Autodesk Inventor part; units mm, degrees
ref_plane "YZ Plane" through (0, 0, 0) normal (1, 0, 0) x (0, 1, 0)
ref_plane "XZ Plane" through (0, 0, 0) normal (0, 1, 0) x (-1, 0, 0)
ref_plane "XY Plane" through (0, 0, 0) normal (0, 0, 1) x (1, 0, 0)
sketch "Skizze1" plane through (0, 0, 0) normal (0, 0, 1) x (1, 0, 0)
  line L0 (21, -21) -> (-21, -21)
  line L1 (-21, -21) -> (-21, 21)
  line L2 (-21, 21) -> (21, 21)
  line L3 (21, 21) -> (21, -21)
  line L4 (21, -21) -> (-21, 21) construction
  line L5 (-21, -21) -> (21, 21) construction
  circle A0 centre (0, 0) radius 18
  circle A1 centre (-15.5, 15.5) radius 1.6
  circle A2 centre (15.5, 15.5) radius 1.6
  circle A3 centre (15.5, -15.5) radius 1.6
  circle A4 centre (-15.5, -15.5) radius 1.6
  dimension "d0" = 42
  dimension "d1" = 42
  dimension "d2" = 36
  dimension "d3" = 31
  dimension "d4" = 15.5
  dimension "d5" = 3.2
  dimension "d6" = 3.2
  dimension "d7" = 3.2
  dimension "d8" = 3.2
extrude "Extrusion1" add sketch "Skizze1" along normal blind 20
sketch "Skizze2" plane through (21, -21, 0) normal (1, 0, 0) x (0, 0, -1)
  line L0 (-25, -16) -> (5, -16)
  line L1 (5, -16) -> (5, 58)
  line L2 (5, 58) -> (-25, 58)
  line L3 (-25, 58) -> (-25, -16)
  line L4 (-25, -16) -> (5, 58) construction
  line L5 (5, -16) -> (-25, 58) construction
  line L6 (0, 0) -> (-20, 0)
  line L7 (0, 42) -> (-20, 42)
  line L8 (0, 42) -> (0, 0)
  point P0 (0, 21)
  point P1 (-10, 21)
  point P2 (0, 21)
  dimension "d11" = 30
  dimension "d12" = 74
  dimension "d13" = 42
  dimension "d14" = 20
  dimension "d15" = 10
  dimension "d16" = 21
extrude "Extrusion2" add sketch "Skizze2" along normal blind 4
sketch "Skizze3" plane through (21, -21, 0) normal (-1, 0, 0) x (0, 0, 1)
  line L0 (0, 0) -> (20, 0)
  line L1 (25, -16) -> (-5, -16)
  line L2 (25, 58) -> (25, -16)
  point P0 (0, 21)
  point P1 (10, -8)
  dimension "d19" = 16
  dimension "d20" = 15
  dimension "d21" = 30
  dimension "d22" = 8
hole "Bohrung1" at (21, -29, 10) direction (1, 0, 0) diameter 5.5 end through all counterbore diameter 15 counterbore depth 1
ref_plane "Arbeitsebene1" through (21, 0, -5) normal (0, -1, 0) x (0, 0, -1)
mirror "Spiegeln1" about plane through (21, 0, -5) normal (0, -1, 0) of "Bohrung1"
chamfer "Fase1" distance 4 angle 45 2 edges at (-21, -21, 10) (-21, 21, 10)
fillet "Rundung1" radius 2 4 edges at (21, 0, 20) (21, -21, 10) (21, 21, 10) (21, 0, 0)
fillet "Rundung2" radius 3 2 edges at (21, -37, 10) (21, 37, 10)
chamfer "Fase2" distance 1 angle 45 10 edges at (21, 0, 25) (21.8787, -36.1213, 25) (24.5, -37, 25) (21.8787, 36.1213, 25) (24.5, 37, 25) (21, 0, -5) (21.8787, 36.1213, -5) (24.5, 37, -5) (21.8787, -36.1213, -5) (24.5, -37, -5)
chamfer "Fase3" distance 1 angle 45 2 edges at (-18, 0, 20) (-18, 0, 0)
equation "\"d1\" = d0"
equation "\"d6\" = d5"
properties part number "bullog_mount"
Can you work these out from the model? Positions are in its coordinate system, mm. A direction names the side the tool comes from. Coordinates: 2 decimals unless noted, no trailing zeros. Loops run counter-clockwise (first coordinate to the right, second up) from the corner with the lowest first, then second, coordinate; pieces in that order, holes last. Notation, with made-up numbers: (9, 17.25) - (53, 17.25) arc R22 cw to (53, 46.25) - close; hole circle Ø2 at (69, 37). An arc over 180 degrees is marked (long way). Answer as a JSON object with one key per item and string values. Group by question number.
Item 1: If we section it at D-D (x = 15.5): State how many separate pieces and enclosed holes the cut face has, plus the area to 3 significant figures.
Item 2: If we section it at C-C (z = 6.5): List the corners of the cut face in (x, y) for me.
Item 3: For pin 1 (4 mm diameter, centred on x = 17.5, z = 11.5, fed in from +Y); pin 2 (4.5 mm diameter, centred on y = 26.5, z = 13, fed in from -X); pin 3 (1.5 mm diameter, centred on x = -4, z = -0.5, fed in from -Y), each with a flat end and sliding along its axis, tell me the tip position at first contact or that it passes through.
Item 4: If I drill on L1, parallel to Y at x = 15.5, z = 12.5; L2, parallel to X at y = -25.5, z = 0.5; L3, parallel to X at y = 26, z = 9.25, over which ranges is the centre line in solid material (lowest first)? Write a range as from..to.
Item 5: On a 3-axis mill with a long thin cutter (end or side, diameter ignored), from which of +Z, -Z, +X, -X, +Y, -Y can I reach the whole of each face in a straight line? I mean faces 1 (the face through (21, 8, 22.5)), 2 (the face through (-19, 3, 0)), 3 (the face through (1, -21, 10)), 4 (the face through (23.521, -31.727, 9.642)), 5 (the face through (22, -29, 13)). Say none if no direction works.
Item 6: If we section it at B-B (y = 29): List the corners of the cut face in (x, z) for me, plus the area to 3 significant figures.
Item 7: If we mould it in two halves opening along X, with no side actions, what happens to faces 6 (the face through (1, 21, 10)), 7 (the face through (25, 1, 10)), 8 (the face through (-16.68, -16.58, 9.86)), 9 (the face through (22.252, -36.438, 10.196))? For each: released by +X, released by -X, zero draft, split by the parting line, or undercut.
Returned:
{
 "1": {"separate pieces": "4", "enclosed holes": "0", "area": "342 mm²"},
 "2": {"outline": "(-21, -17) - (-17, -21) - (19, -21) arc R2 cw to (20.9, -22.37) - (22, -22.37) - (22, -35.63) - (21.48, -35.63) arc R3 ccw to (24, -37) - (25, -37) - (25, 37) - (24, 37) arc R3 ccw to (21.48, 35.63) - (22, 35.63) - (22, 22.37) - (20.9, 22.37) arc R2 cw to (19, 21) - (-17, 21) - (-21, 17) - close; hole circle Ø36 at (0, 0); hole circle Ø3.2 at (-15.5, -15.5); hole circle Ø3.2 at (-15.5, 15.5); hole circle Ø3.2 at (15.5, -15.5); hole circle Ø3.2 at (15.5, 15.5)"},
 "3": {"pin 1": "stops at y = 21.06", "pin 2": "stops at x = 22", "pin 3": "stops at y = -21"},
 "4": {"L1": "y = -21..-17.1, -13.9..-9.15, 9.15..13.9, 17.1..21", "L2": "x = 21..25", "L3": "x = 22..25"},
 "5": {"face 1": "+Z, -X", "face 2": "-Z, -X, +Y, -Y", "face 3": "+Z, -Z, -X, -Y", "face 4": "+X, -X", "face 5": "-X"},
 "6": {"outline": "(21, -4) - (22, -5) - (25, -5) - (25, 7.25) - (22, 7.25) - (22, 2.5) - (21, 2.5) - close; (21, 17.5) - (22, 17.5) - (22, 12.75) - (25, 12.75) - (25, 25) - (22, 25) - (21, 24) - close", "area": "87.5 mm²"},
 "7": {"face 6": "zero draft", "face 7": "released by +X", "face 8": "undercut", "face 9": "released by -X"}
}
